Geometry: final body of the model. Coordinates: model frame, mm. A direction names the side the tool comes from. Give positions to 0.01 mm unless a question says otherwise; leave off trailing zeros. Loops run counter-clockwise (first coordinate to the right, second up) from the corner with the lowest first, then second, coordinate; pieces in that order, holes last.
1. Section A-A, the plane y = 0. Output: boundary loops of the cut face in (x, z), then the cut area to 3 significant figures.
2. Draft query along Y for faces 1 (the face through (72, 48, 9)), 2 (the face through (7.5, 61, 2)), 3 (the face through (-4.686, 35.694, 0.986)). Return one class per face: +Y half, -Y half, draft (parallel to the pull), parting line (faces both ways), or undercut.
3. First-contact query: P1, Ø3, axis at y = 13.5, z = 5, coming from the +X side; P2, Ø3.5, axis at x = 57.5, z = 8, coming from the -Y side; P3, Ø10, axis at x = 59, y = 30.5, coming from the -Z side. Flat tips, straight axial feed; report the tip coordinate or a pass-through.
4. Access query for faces 4 (the face through (63, 30, 7)), 5 (the face through (-63, 30, 7)), 6 (the face through (0, 65, 5)), 7 (the face through (-51.5, -1, 6)). Directions: +Z, -Z, +X, -X, +Y, -Y. A direction counts if a zero-diameter tool reaches every point of the face in a straight line with its end or side. Return the directions, or none.
5. Section C-C, the plane z = 8.5. Output: boundary loops of the cut face in (x, y).
6. Section B-B, the plane x = -12. Output: boundary loops of the cut face in (y, z).
7. Material intervals for line 1 along Y through (x, z) = (0, 3.45); line 2 along Y through (x, z) = (0, 1.3); line 3 along Y through (x, z) = (-39, 8.75), sorted ascending.
from build123d import *

# Parameters (mm, degrees)
F0_W      = 103
F0_H      = 103
F1_DEPTH  = 10
F0_R      = 36
F2_DEPTH  = 2
F0_R_2    = 1.5
F4_DEPTH  = 5
F3_W      = 10
F3_H      = 4
F5_DEPTH  = 25
F6_W      = 10
F6_H      = 4
F7_DEPTH  = 25
F8_W      = 2
F8_H      = 10
F9_DEPTH  = 17
F11_DEPTH = 2
F13_DEPTH = 2
F14_R     = 1.25
F15_DEPTH = 3.5
F16_R     = 1.25
F17_DEPTH = 3.5
F19_DEPTH = 3


with BuildPart() as f1:
    # F0 (on Top) → F1 (new body)
    with BuildSketch(Plane.XY):
        Polygon((53, -53), (53, 53), (7.5, 53), (-7.5, 53), (-53, 53), (-53, -53), align=None)
        Rectangle(F0_W, F0_H, mode=Mode.SUBTRACT)
    extrude(amount=F1_DEPTH)

    # F0 (on Top) → F2 (join)
    with BuildSketch(Plane.XY):
        Rectangle(F0_W, F0_H)
        Circle(F0_R, mode=Mode.SUBTRACT)
    extrude(amount=F2_DEPTH)

    # F0 (on Top) → F4 (join)
    with BuildSketch(Plane.XY):
        Polygon((53, -53), (53, 53), (7.5, 53), (-7.5, 53), (-53, 53), (-53, -53), align=None)
        Rectangle(F0_W, F0_H, mode=Mode.SUBTRACT)
        with BuildLine():
            Line((-7.5, 53), (7.5, 53))
            Line((7.5, 53), (7.5, 70))
            ThreePointArc((7.5, 70), (0, 77.5), (-7.5, 70))
            Line((-7.5, 70), (-7.5, 53))
        make_face()
        with Locations((0, 70)):
            Circle(F0_R_2, mode=Mode.SUBTRACT)
    extrude(amount=F4_DEPTH)

    # F3 (on face) → F5 (cut)
    with BuildSketch(Plane.YZ.offset(-51.5)):
        with Locations((31.5, 4)):
            Rectangle(F3_W, F3_H)
        with Locations((-31.5, 4)):
            Rectangle(F3_W, F3_H)
    extrude(amount=-F5_DEPTH, mode=Mode.SUBTRACT)

    # F6 (on face) → F7 (cut)
    with BuildSketch(Plane(origin=(51.5, 0, 0), x_dir=(0, -1, 0), z_dir=(-1, 0, 0))):
        with Locations((-31.5, 4)):
            Rectangle(F6_W, F6_H)
        with Locations((31.5, 4)):
            Rectangle(F6_W, F6_H)
    extrude(amount=-F7_DEPTH, mode=Mode.SUBTRACT)

    # F8 (on face) → F9 (join)
    with BuildSketch(Plane.XZ.offset(53)):
        with Locations((-52, 5)):
            Rectangle(F8_W, F8_H)
        with Locations((52, 5)):
            Rectangle(F8_W, F8_H)
    extrude(amount=F9_DEPTH)

    # F10 (on face) → F11 (join)
    with BuildSketch(Plane(origin=(-53, 0, 0), x_dir=(0, -1, 0), z_dir=(-1, 0, 0))):
        with BuildLine():
            Line((70, 10), (70, 0))
            ThreePointArc((70, 0), (75, 5), (70, 10))
        make_face()
    extrude(amount=-F11_DEPTH)

    # F12 (on face) → F13 (join)
    with BuildSketch(Plane.YZ.offset(53)):
        with BuildLine():
            Line((-70, 0), (-70, 10))
            ThreePointArc((-70, 10), (-75, 5), (-70, 0))
        make_face()
    extrude(amount=-F13_DEPTH)

    # F14 (on face) → F15 (join)
    with BuildSketch(Plane.YZ.offset(-51)):
        with Locations((-70, 5)):
            Circle(F14_R)
    extrude(amount=F15_DEPTH)

    # F16 (on face) → F17 (join)
    with BuildSketch(Plane(origin=(51, 0, 0), x_dir=(0, -1, 0), z_dir=(-1, 0, 0))):
        with Locations((70, 5)):
            Circle(F16_R)
    extrude(amount=F17_DEPTH)

    # F18 (on face) → F19 (join)
    with BuildSketch(Plane.XY.offset(10)):
        with BuildLine():
            Line((68, 50), (53, 50))
            Line((53, 50), (53, 10))
            Line((53, 10), (68, 10))
            ThreePointArc((68, 10), (71.5355339059, 11.4644660941), (73, 15))
            Line((73, 15), (73, 45))
            ThreePointArc((73, 45), (71.5355339059, 48.5355339059), (68, 50))
        make_face()
    extrude(amount=-F19_DEPTH)

    # F20: F1 across plane


with BuildPart() as f1_1:
    add(f1.part)
    add(f1.part.mirror(Plane.YZ))


solid = f1_1.part
Answers below:
1. outline: (-53, 0) - (-36, 0) - (-36, 2) - (-51.5, 2) - (-51.5, 10) - (-53, 10) - close; (36, 0) - (53, 0) - (53, 10) - (51.5, 10) - (51.5, 2) - (36, 2) - close
1. area: 92.0 mm2
2. face 1: +Y half
2. face 2: draft
2. face 3: undercut
3. P1: stops at x = 53
3. P2: stops at y = 10
3. P3: stops at z = 7
4. face 4: -Z, +X, +Y, -Y
4. face 5: -Z, -X, +Y, -Y
4. face 6: +Z, +X, -X, +Y
4. face 7: +Z
5. outline: (-73, 15) arc R5 ccw to (-68, 10) - (-53, 10) - (-53, -73.57) - (-51, -73.57) - (-51, -53) - (51, -53) - (51, -73.57) - (53, -73.57) - (53, 10) - (68, 10) arc R5 ccw to (73, 15) - (73, 45) arc R5 ccw to (68, 50) - (53, 50) - (53, 53) - (-53, 53) - (-53, 50) - (-68, 50) arc R5 ccw to (-73, 45) - close; hole (-51.5, -51.5) - (51.5, -51.5) - (51.5, 51.5) - (-51.5, 51.5) - close
6. outline: (-53, 0) - (-33.94, 0) - (-33.94, 2) - (-51.5, 2) - (-51.5, 10) - (-53, 10) - close; (33.94, 0) - (53, 0) - (53, 10) - (51.5, 10) - (51.5, 2) - (33.94, 2) - close
7. line 1: y = -53 to -51.5, 51.5 to 68.5, 71.5 to 77.5
7. line 2: y = -53 to -36, 36 to 68.5, 71.5 to 77.5
7. line 3: y = -53 to -51.5, 51.5 to 53
